For this review, take the finished solid that the model builds, in its own axes (mm). A direction names the side the tool comes from. Coordinates: 2 decimals unless noted, no trailing zeros. Loops run counter-clockwise (first coordinate to the right, second up) from the corner with the lowest first, then second, coordinate; pieces in that order, holes last.
1. Take a section at B-B, the plane z = 10. State the section outline as (x, y) points, then the cut area to 3 significant figures.
2. Take a section at C-C, the plane x = -10. State the section outline as (y, z) points, then the cut area to 3 significant figures.
3. To check wall thickness, follow probe 1 along X at (y, z) = (5, 15.5); probe 2 along X at (y, z) = (17, 2.5); probe 3 along Y at (x, z) = (11.5, 6). State the ranges of each line that lie inside material, in increasing order.
4. Clearance check with flat-ended pins moving along their axes: P1, Ø3, axis at y = 18, z = 10, coming from the -X side; P2, Ø5, axis at x = -7.5, z = 18, coming from the -Y side; P3, Ø2, axis at x = 4, z = 4.5, coming from the +Y side; P4, Ø1.4, axis at x = -10, z = 8, coming from the -Y side. State where each tip first meets the part, or that it passes through.
5. Mouldability with a two-part tool opening along Z and no side actions: class faces 1 (the face through (12.398, 23.537, 6.202)), 2 (the face through (10, 8, 0)), 3 (the face through (0, -14, 10)), 4 (the face through (10, 8, 20)) as pulls with the +Z half, pulls with the -Z half, needs draft (parallel to the pull), parting line crosses it, or undercut.
6. Machinability: for faces 5 (the face through (14, 15, 10)), 6 (the face through (10, 25, 10)), 7 (the face through (9, 7, 10)), which of the approach directions +Z, -Z, +X, -X, +Y, -Y give a long, thin tool a straight path to every point of the face, cutting with its end or side? Answer none if there is none.
7. Take a section at D-D, the plane z = 1.75. State the section outline as (x, y) points.
8. Take a section at A-A, the plane y = 24.5. State the section outline as (x, z) points.
```python
from build123d import *

# Parameters (mm, degrees)
EXTRUDE_1_DEPTH     = 20
SKETCH_2_R          = 1.55
CUT_EXTRUDE_1_DEPTH = 30
SKETCH_3_W          = 1.75
SKETCH_3_H          = 10
CUT_EXTRUDE_2_DEPTH = 20


with BuildPart() as part:
    # 草图1 → 凸台-拉伸1 (new body)
    with BuildSketch(Plane.XY):
        with BuildLine():
            Line((-14, 0), (-14, 30))
            Line((-14, 30), (-9, 30))
            Line((-9, 30), (-9, 0))
            ThreePointArc((-9, 0), (0, -9), (9, 0))
            Line((9, 0), (9, 30))
            Line((9, 30), (14, 30))
            Line((14, 30), (14, 0))
            ThreePointArc((14, 0), (0, -14), (-14, 0))
        make_face()
    extrude(amount=EXTRUDE_1_DEPTH)

    # 草图2 → 切除-拉伸1 (cut)
    with BuildSketch(Plane(origin=(14, 0, 0), x_dir=(0, 0, -1), z_dir=(1, 0, 0))):
        with Locations((-10, 18)):
            Circle(SKETCH_2_R)
        with Locations((-6, 22)):
            Circle(SKETCH_2_R)
    extrude(amount=-CUT_EXTRUDE_1_DEPTH, mode=Mode.SUBTRACT)

    # 草图3 → 切除-拉伸2 (cut)
    with BuildSketch(Plane(origin=(0, 0, 0), x_dir=(-1, 0, 0), z_dir=(0, 0, -1))):
        with Locations((-9.875, 20)):
            Rectangle(SKETCH_3_W, SKETCH_3_H)
    cut_extrude_2 = extrude(amount=-CUT_EXTRUDE_2_DEPTH, mode=Mode.SUBTRACT)

    # 镜向1: 切除-拉伸2 across plane
    add(cut_extrude_2.mirror(Plane(origin=(0, 0, 0), x_dir=(0, 0, 1), z_dir=(1, 0, 0))), mode=Mode.SUBTRACT)


solid = part.part
```
Results list:
1. outline: (-14, 0) arc R14 ccw to (14, 0) - (14, 16.45) - (10.75, 16.45) - (10.75, 15) - (9, 15) - (9, 0) arc R9 cw to (-9, 0) - (-9, 15) - (-10.75, 15) - (-10.75, 16.45) - (-14, 16.45) - close; (-14, 19.55) - (-10.75, 19.55) - (-10.75, 25) - (-9, 25) - (-9, 30) - (-14, 30) - close; (9, 25) - (10.75, 25) - (10.75, 19.55) - (14, 19.55) - (14, 30) - (9, 30) - close
1. area: 425 mm2
2. outline: (-9.8, 0) - (15, 0) - (15, 20) - (-9.8, 20) - close; (25, 0) - (30, 0) - (30, 20) - (25, 20) - close
2. area: 596 mm2
3. probe 1: x = -14 to -9, 9 to 14
3. probe 2: x = -14 to -10.75, 10.75 to 14
3. probe 3: y = -7.98 to 20.45, 23.55 to 30
4. P1: passes through
4. P2: stops at y = -13.08
4. P3: stops at y = -7.48
4. P4: stops at y = -10.46
5. face 1: undercut
5. face 2: pulls with the -Z half
5. face 3: needs draft
5. face 4: pulls with the +Z half
6. face 5: +Z, -Z, +X, +Y, -Y
6. face 6: +Z, -Z
6. face 7: +Z, -Z, +Y
7. outline: (-14, 0) arc R14 ccw to (14, 0) - (14, 30) - (9, 30) - (9, 25) - (10.75, 25) - (10.75, 15) - (9, 15) - (9, 0) arc R9 cw to (-9, 0) - (-9, 15) - (-10.75, 15) - (-10.75, 25) - (-9, 25) - (-9, 30) - (-14, 30) - close
8. outline: (-14, 0) - (-10.75, 0) - (-10.75, 20) - (-14, 20) - close; (10.75, 0) - (14, 0) - (14, 20) - (10.75, 20) - close
